Check sheet for the modelled part. Datum: model origin and axes. Units: mm. A direction names the side the tool comes from. Give positions to 0.01 mm unless a question says otherwise; leave off trailing zeros. Write each loop counter-clockwise with the first axis right and the second up, starting at its lowest first coordinate (ties: lowest second). Pieces come first, ordered by that corner, then holes. Notation, with made-up numbers: M 71.5,4 L 105.5,4 A21 cw 105.5,14 Z; hole C -21.5,-34 d10. An arc over 180 degrees is marked long. One line per item, written item: value. Start each with the question number.
from build123d import *

# Parameters (mm, degrees)
SKETCH2_W           = 45.7
SKETCH2_H           = 15
BOSS_EXTRUDE1_DEPTH = 10
SKETCH4_R           = 3
CUT_EXTRUDE1_DEPTH  = 50.127283662
SKETCH5_W           = 15
SKETCH5_H           = 10
CUT_EXTRUDE2_DEPTH  = 5
CHAMFER1_SIZE       = 4.990232455
CHAMFER1_SIZE_2     = 13
CHAMFER2_SIZE       = 0.965614075


with BuildPart() as part:
    # Sketch2 → Boss-Extrude1 (new body)
    with BuildSketch(Plane(origin=(0, 0, 0), x_dir=(1, 0, 0), z_dir=(0, 1, 0))):
        with Locations((-22.85, -7.5)):
            Rectangle(SKETCH2_W, SKETCH2_H)
    extrude(amount=BOSS_EXTRUDE1_DEPTH)

    # Sketch3 → Cut-Revolve1 (revolve, cut)
    with BuildSketch(Plane(origin=(0, 0, 0), x_dir=(-1, 0, 0), z_dir=(0, 0, -1))):
        with BuildLine():
            Line((22.85, 14), (22.85, -4))
            ThreePointArc((22.85, -4), (13.85, 5), (22.85, 14))
        make_face()
    revolve(axis=Axis((-22.85, 14, 0), (0, -1, 0)), mode=Mode.SUBTRACT)

    # Sketch4 → Cut-Extrude1 (cut, through all)
    with BuildSketch(Plane(origin=(0, 0, 0), x_dir=(-1, 0, 0), z_dir=(0, 0, -1))):
        with Locations((6.5, 5)):
            Circle(SKETCH4_R)
        with Locations((39.2, 5)):
            Circle(SKETCH4_R)
    extrude(amount=-CUT_EXTRUDE1_DEPTH, mode=Mode.SUBTRACT)

    # Sketch5 → Cut-Extrude2 (cut)
    with BuildSketch(Plane.XY.offset(15)):
        with Locations((-38.2, 5)):
            Rectangle(SKETCH5_W, SKETCH5_H)
        with Locations((-7.5, 5)):
            Rectangle(SKETCH5_W, SKETCH5_H)
    extrude(amount=-CUT_EXTRUDE2_DEPTH, mode=Mode.SUBTRACT)

    # Chamfer1
    # the kernel refuses this chamfer: 13, 4.990232455 mm, written as the material it takes off along each edge
    with BuildSketch(Plane(origin=(-15, 43.716873314, 15), x_dir=(0, 0, -1), z_dir=(0, -1, 0))) as chamfer1_piece_1:
        Polygon((CHAMFER1_SIZE, 0), (0, -CHAMFER1_SIZE_2), (0, 0), align=None)
    extrude(amount=77.433746627, mode=Mode.SUBTRACT)
    with BuildSketch(Plane(origin=(-30.7, 43.716873314, 15), x_dir=(1, 0, 0), z_dir=(0, -1, 0))) as chamfer1_piece_2:
        Polygon((CHAMFER1_SIZE_2, 0), (0, -CHAMFER1_SIZE), (0, 0), align=None)
    extrude(amount=77.433746627, mode=Mode.SUBTRACT)

    # Chamfer2
    # the kernel refuses this chamfer: 1, 0.965614075 mm, written as the material it takes off along each edge
    with BuildSketch(Plane(origin=(-22.85, 0, 0), x_dir=(-0.9379115380464662, 0, -0.34687454043113636), z_dir=(0.34687454043113636, 0, -0.9379115380464662))) as chamfer2_piece_1:
        with BuildLine():
            Line((7.483314774 + CHAMFER2_SIZE, 0), (8.008407714, 0.893248743))
            ThreePointArc((8.008407714, 0.893248743), (7.764305072, 0.44856432), (7.483314774, 0))
            Line((7.483314774, 0), (7.483314774 + CHAMFER2_SIZE, 0))
        make_face()
    revolve(axis=Axis((-22.85, 0, 0), (0, 1, 0)), revolution_arc=220.592533512, mode=Mode.SUBTRACT)
    with BuildSketch(Plane(origin=(-22.85, 10, 0), x_dir=(-0.9379115380464663, 0, -0.3468745404311359), z_dir=(0.3468745404311359, 0, -0.9379115380464663))) as chamfer2_piece_2:
        with BuildLine():
            Line((8.008407714, -0.893248743), (7.483314774 + CHAMFER2_SIZE, 0))
            Line((7.483314774 + CHAMFER2_SIZE, 0), (7.483314774, 0))
            ThreePointArc((7.483314774, 0), (7.764305072, -0.44856432), (8.008407714, -0.893248743))
        make_face()
    revolve(axis=Axis((-22.85, 10, 0), (0, 1, 0)), revolution_arc=220.592533512, mode=Mode.SUBTRACT)


solid = part.part
1) Cross-section at D-D (x = -7). Record the boundary of the cut face in (y, z), plus the area to 3 significant figures.
2) Cross-section at B-B (x = -39.2). Record the boundary of the cut face in (y, z).
3) Material ranges on L1, parallel to Y at x = -39.2, z = 8; L2, parallel to X at y = 7.5, z = 4; L3, parallel to X at y = 2.25, z = 9.5, recorded low to high. Write a range as from..to.
4) Tool access check on faces 4 (the flat face through (-36.6, 7.3, 10)), 5 (the flat face through (-9, 7, 10)), 6 (the flat face through (-23, 0, 9)). Record the directions out of +Z, -Z, +X, -X, +Y, -Y that give a thin tool (end or side, any length) a straight path to the whole face; none if there is none.
5) Cross-section at A-A (y = 5). State how many separate pieces and enclosed holes the cut face has, plus the area to 3 significant figures.
6) Gauge pin test, flat end, axial feed: pin 1 (1 mm diameter, centred on x = -19.5, y = 3.5, fed in from -Z). Record the tip position at first contact, or that the pin passes through.
7) Draft check along Y on faces 1 (the flat face through (-23, 10, 9)), 2 (the cylindrical face through (-36.2, 5.1, 4.9)), 3 (the flat face through (0, 5, 5)). Enter one of: released by +Y, released by -Y, zero draft, split by the parting line, or undercut.
Data:
1. outline: M 0,0 L 2.04,0 L 2.04,10 L 0,10 Z; M 7.96,0 L 10,0 L 10,10 L 7.96,10 Z
1. area: 40.8 mm2
2. outline: M 0,0 L 2,0 L 2,10 L 0,10 Z; M 8,0 L 10,0 L 10,10 L 8,10 Z
3. L1: y = 0..2, 8..10
3. L2: x = -45.7..-40.86, -37.54..-30.51, -15.19..-8.16, -4.84..0
3. L3: x = -45.7..-40.4, -38..-7.7, -5.3..0
4. face 4: +Z, -X, +Y, -Y
4. face 5: +Z, +X, +Y, -Y
4. face 6: +Z, -Z, +X, -X, -Y
5. separate pieces: 3
5. enclosed holes: 0
5. area: 234 mm2
6. pin 1: stops at z = 7.98
7. face 1: released by +Y
7. face 2: undercut
7. face 3: zero draft
